Could you check a few things on this model? Use its own coordinates, in mm. Face numbers are marked on the shaded views. Round coordinates to 2 decimals unless told otherwise and drop trailing zeros. Loops run counter-clockwise (first coordinate to the right, second up) from the corner with the lowest first, then second, coordinate; pieces in that order, holes last. Notation, with made-up numbers: (-11.5, 0.25) -> (24.5, 0.25) arc R34 cw to (24.5, 36.25) -> close; hole circle Ø9 at (50, 9). An arc over 180 degrees is marked (long way). Write each question's results on one line, items separated by ' | '.
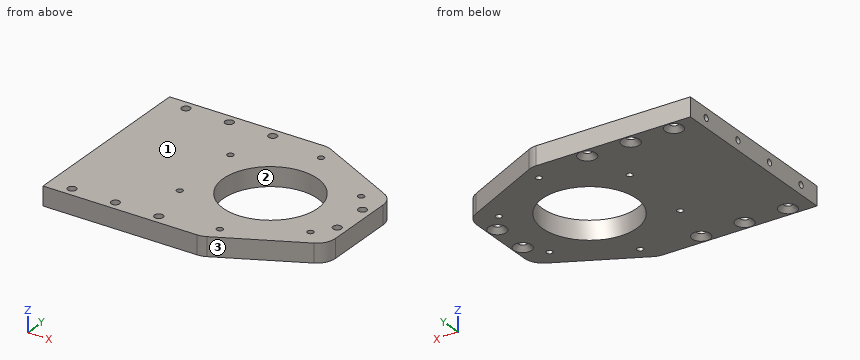
from build123d import *

# Parameters (mm, degrees)
EXTRUDE1_DEPTH                                  = 10
SKETCH5_R                                       = 25
CUT_EXTRUDE1_DEPTH                              = 20
SKETCH6_R                                       = 1.65
CUT_EXTRUDE2_DEPTH                              = 15
CUT_EXTRUDE3_REACH                              = 145.467
SKETCH7_R                                       = 1.5
CSK_FOR_M4_FLAT_HEAD_MACHINE_SCREW1_D           = 4.5
CSK_FOR_M4_FLAT_HEAD_MACHINE_SCREW1_CSINK_D     = 9.4
CSK_FOR_M4_FLAT_HEAD_MACHINE_SCREW1_CSINK_ANGLE = 90
SKETCH10_R                                      = 1.65
CUT_EXTRUDE4_DEPTH                              = 10
FILLET1_R                                       = 10
SKETCH13_R                                      = 2.25
CUT_EXTRUDE5_DEPTH                              = 10
CSK_FOR_M4_FLAT_HEAD_MACHINE_SCREW3_D           = 4.5
CSK_FOR_M4_FLAT_HEAD_MACHINE_SCREW3_CSINK_D     = 9.4
CSK_FOR_M4_FLAT_HEAD_MACHINE_SCREW3_CSINK_ANGLE = 90


with BuildPart() as part:
    # Sketch1 → Extrude1 (new body)
    with BuildSketch(Plane.XY):
        Polygon((0, -50), (84.1, -50), (134.1, -25), (134.1, 25), (84.1, 50), (0, 50), align=None)
    extrude(amount=EXTRUDE1_DEPTH)

    # Sketch5 → Cut-Extrude1 (cut)
    with BuildSketch(Plane.XY.offset(10)):
        with Locations((87, 0)):
            Circle(SKETCH5_R)
    extrude(amount=-CUT_EXTRUDE1_DEPTH, mode=Mode.SUBTRACT)

    # Sketch6 → Cut-Extrude2 (cut)
    with BuildSketch(Plane.ZY):
        with Locations((5, 37.5)):
            Circle(SKETCH6_R)
        with Locations((5, 12.5)):
            Circle(SKETCH6_R)
        with Locations(Location((5, -37.5, 0), (0, 0, 180))):
            Circle(SKETCH6_R)
        with Locations(Location((5, -12.5, 0), (0, 0, 180))):
            Circle(SKETCH6_R)
    extrude(amount=-CUT_EXTRUDE2_DEPTH, mode=Mode.SUBTRACT)

    # Sketch7 → Cut-Extrude3 (cut, up to next)
    with BuildSketch(Plane(origin=(0, 0, 0), x_dir=(-1, 0, 0), z_dir=(0, 0, -1)), mode=Mode.PRIVATE) as cut_extrude3_sk1:
        with Locations((-12, 45)):
            Circle(SKETCH7_R)
    cut_extrude3_tool1 = extrude(cut_extrude3_sk1.sketch, amount=-CUT_EXTRUDE3_REACH, mode=Mode.PRIVATE) & part.part
    # Sketch7 → Cut-Extrude3 (cut, up to next)
    with BuildSketch(Plane(origin=(0, 0, 0), x_dir=(-1, 0, 0), z_dir=(0, 0, -1)), mode=Mode.PRIVATE) as cut_extrude3_sk2:
        with Locations(Location((-35, 45, 0), (0, 0, 180))):
            Circle(SKETCH7_R)
    cut_extrude3_tool2 = extrude(cut_extrude3_sk2.sketch, amount=-CUT_EXTRUDE3_REACH, mode=Mode.PRIVATE) & part.part
    # Sketch7 → Cut-Extrude3 (cut, up to next)
    with BuildSketch(Plane(origin=(0, 0, 0), x_dir=(-1, 0, 0), z_dir=(0, 0, -1)), mode=Mode.PRIVATE) as cut_extrude3_sk3:
        with Locations(Location((-58, 45, 0), (0, 0, 180))):
            Circle(SKETCH7_R)
    cut_extrude3_tool3 = extrude(cut_extrude3_sk3.sketch, amount=-CUT_EXTRUDE3_REACH, mode=Mode.PRIVATE) & part.part
    # Sketch7 → Cut-Extrude3 (cut, up to next)
    with BuildSketch(Plane(origin=(0, 0, 0), x_dir=(-1, 0, 0), z_dir=(0, 0, -1)), mode=Mode.PRIVATE) as cut_extrude3_sk4:
        with Locations((-58, -45)):
            Circle(SKETCH7_R)
    cut_extrude3_tool4 = extrude(cut_extrude3_sk4.sketch, amount=-CUT_EXTRUDE3_REACH, mode=Mode.PRIVATE) & part.part
    # Sketch7 → Cut-Extrude3 (cut, up to next)
    with BuildSketch(Plane(origin=(0, 0, 0), x_dir=(-1, 0, 0), z_dir=(0, 0, -1)), mode=Mode.PRIVATE) as cut_extrude3_sk5:
        with Locations((-35, -45)):
            Circle(SKETCH7_R)
    cut_extrude3_tool5 = extrude(cut_extrude3_sk5.sketch, amount=-CUT_EXTRUDE3_REACH, mode=Mode.PRIVATE) & part.part
    # Sketch7 → Cut-Extrude3 (cut, up to next)
    with BuildSketch(Plane(origin=(0, 0, 0), x_dir=(-1, 0, 0), z_dir=(0, 0, -1)), mode=Mode.PRIVATE) as cut_extrude3_sk6:
        with Locations(Location((-12, -45, 0), (0, 0, 180))):
            Circle(SKETCH7_R)
    cut_extrude3_tool6 = extrude(cut_extrude3_sk6.sketch, amount=-CUT_EXTRUDE3_REACH, mode=Mode.PRIVATE) & part.part
    add(cut_extrude3_tool1.solids().sort_by_distance((12, 45, 0))[0], mode=Mode.SUBTRACT)
    add(cut_extrude3_tool2.solids().sort_by_distance((35, 45, 0))[0], mode=Mode.SUBTRACT)
    add(cut_extrude3_tool3.solids().sort_by_distance((58, 45, 0))[0], mode=Mode.SUBTRACT)
    add(cut_extrude3_tool4.solids().sort_by_distance((58, -45, 0))[0], mode=Mode.SUBTRACT)
    add(cut_extrude3_tool5.solids().sort_by_distance((35, -45, 0))[0], mode=Mode.SUBTRACT)
    add(cut_extrude3_tool6.solids().sort_by_distance((12, -45, 0))[0], mode=Mode.SUBTRACT)

    # CSK for M4 Flat Head Machine Screw1 (through all)
    with Locations(Plane(origin=(0, 0, 0), x_dir=(-1, 0, 0), z_dir=(0, 0, -1))):
        with Locations((-12, 45), (-35, 45), (-58, 45), (-12, -45), (-35, -45), (-58, -45)):
            CounterSinkHole(CSK_FOR_M4_FLAT_HEAD_MACHINE_SCREW1_D / 2, CSK_FOR_M4_FLAT_HEAD_MACHINE_SCREW1_CSINK_D / 2, counter_sink_angle=CSK_FOR_M4_FLAT_HEAD_MACHINE_SCREW1_CSINK_ANGLE)

    # Sketch10 → Cut-Extrude4 (cut)
    with BuildSketch(Plane(origin=(0, 0, 0), x_dir=(-1, 0, 0), z_dir=(0, 0, -1))):
        with Locations((-87, 40)):
            Circle(SKETCH10_R)
        with Locations((-52.358983849, 20)):
            Circle(SKETCH10_R)
        with Locations((-52.358983849, -20)):
            Circle(SKETCH10_R)
        with Locations((-87, -40)):
            Circle(SKETCH10_R)
        with Locations((-121.641016151, -20)):
            Circle(SKETCH10_R)
        with Locations((-121.641016151, 20)):
            Circle(SKETCH10_R)
    extrude(amount=-CUT_EXTRUDE4_DEPTH, mode=Mode.SUBTRACT)

    # Fillet1
    fillet1_edges = [part.edges().sort_by_distance(p)[0] for p in [
        (84.1, 50, 5),
        (134.1, 25, 5),
        (134.1, -25, 5),
        (84.1, -50, 5),
    ]]
    fillet(fillet1_edges, radius=FILLET1_R)

    # Sketch13 → Cut-Extrude5 (cut)
    with BuildSketch(Plane(origin=(0, 0, 0), x_dir=(-1, 0, 0), z_dir=(0, 0, -1))):
        with Locations((-129.1, 10)):
            Circle(SKETCH13_R)
        with Locations(Location((-129.1, -10, 0), (0, 0, 180))):
            Circle(SKETCH13_R)
    extrude(amount=-CUT_EXTRUDE5_DEPTH, mode=Mode.SUBTRACT)

    # CSK for M4 Flat Head Machine Screw3 (through all)
    with Locations(Plane(origin=(0, 0, 0), x_dir=(-1, 0, 0), z_dir=(0, 0, -1))):
        with Locations((-129.1, 10), (-129.1, -10)):
            CounterSinkHole(CSK_FOR_M4_FLAT_HEAD_MACHINE_SCREW3_D / 2, CSK_FOR_M4_FLAT_HEAD_MACHINE_SCREW3_CSINK_D / 2, counter_sink_angle=CSK_FOR_M4_FLAT_HEAD_MACHINE_SCREW3_CSINK_ANGLE)


solid = part.part
1) I want a section at B-B, the plane x = 12. Write out the boundary of the cut face in (y, z), plus the area to 3 significant figures.
Model answer:
outline: (-50, 0) -> (-49.7, 0) -> (-47.25, 2.45) -> (-47.25, 10) -> (-50, 10) -> close; (-42.75, 2.45) -> (-40.3, 0) -> (40.3, 0) -> (42.75, 2.45) -> (42.75, 10) -> (-42.75, 10) -> close; (47.25, 2.45) -> (49.7, 0) -> (50, 0) -> (50, 10) -> (47.25, 10) -> close; hole circle Ø3.3 at (-37.5, 5); hole circle Ø3.3 at (-12.5, 5); hole circle Ø3.3 at (12.5, 5); hole circle Ø3.3 at (37.5, 5) | area: 864 mm2
2) I'm going to push flat-ended pins straight in: pin 1 (3 mm diameter, centred on y = 37.5, z = 5, fed in from +X); pin 2 (6 mm diameter, centred on x = 12, y = 45, fed in from -Z); pin 3 (1 mm diameter, centred on y = -37.5, z = 4.5, fed in from -X). Where does each tip first touch, or does it pass through?
Model answer:
pin 1: stops at x = 112.1 | pin 2: stops at z = 1.7 | pin 3: stops at x = 15
3) I need wall thicknesses on line 1 (Y direction, x = 35, z = 9.75); line 2 (Y direction, x = 6.5, z = 5); line 3 (X direction, y = -45, z = 8.25). Which ranges of each line are inside material? Lowest first, please.
Model answer:
line 1: y = -50 to -47.25, -42.75 to 42.75, 47.25 to 50 | line 2: y = -50 to -39.15, -35.85 to -14.15, -10.85 to 10.85, 14.15 to 35.85, 39.15 to 50 | line 3: x = 0 to 9.75, 14.25 to 32.75, 37.25 to 55.75, 60.25 to 94.1
4) I want a section at C-C, the plane y = 0. Write out the boundary of the cut face in (x, z), plus the area to 3 significant figures.
Model answer:
outline: (0, 0) -> (62, 0) -> (62, 10) -> (0, 10) -> close; (112, 0) -> (134.1, 0) -> (134.1, 10) -> (112, 10) -> close | area: 841 mm2
5) If we mould it in two halves opening along X, with no side actions, what happens to the marked faces 1, 2 and 3? For each: released by +X, released by -X, zero draft, split by the parting line, or undercut.
Model answer:
face 1: zero draft | face 2: undercut | face 3: released by +X
6) I want a section at A-A, the plane x = 102. Write out the boundary of the cut face in (y, z).
Model answer:
outline: (-41.05, 0) -> (-20, 0) -> (-20, 10) -> (-41.05, 10) -> close; (20, 0) -> (41.05, 0) -> (41.05, 10) -> (20, 10) -> close
7) I want a section at D-D, the plane y = 45. Write out the boundary of the cut face in (x, z), plus the area to 3 significant figures.
Model answer:
outline: (0, 0) -> (7.3, 0) -> (9.75, 2.45) -> (9.75, 10) -> (0, 10) -> close; (14.25, 2.45) -> (16.7, 0) -> (30.3, 0) -> (32.75, 2.45) -> (32.75, 10) -> (14.25, 10) -> close; (37.25, 2.45) -> (39.7, 0) -> (53.3, 0) -> (55.75, 2.45) -> (55.75, 10) -> (37.25, 10) -> close; (60.25, 2.45) -> (62.7, 0) -> (94.1, 0) -> (94.1, 10) -> (60.25, 10) -> close | area: 788 mm2
